Design review of the part built by this model. Coordinates are the model's own, in mm. A direction names the side the tool comes from. Coordinates: 2 decimals unless noted, no trailing zeros. Loops run counter-clockwise (first coordinate to the right, second up) from the corner with the lowest first, then second, coordinate; pieces in that order, holes last. Notation, with made-up numbers: M 34,23 L 75,23 A23 cw 75,34 Z; hole C 6.25,82 d5. An arc over 180 degrees is marked long. Put each result on its own line as item: value. Start each with the question number.
(1) For faces 4 (the cylindrical face through (28.795, 39.415, 2.535)), 5 (the flat face through (173.551, 4.735, 2.465)), list the 3-axis set-ups (+Z, -Z, +X, -X, +Y, -Y) from which the entire face can be reached by the end or side of a thin tool; tool diameter is ignored.
(2) Take a section at B-B, the plane x = 0. Give the boundary of the cut face in (y, z).
(3) Take a section at D-D, the plane y = 0. Give the boundary of the cut face in (x, z).
(4) Clearance check with flat-ended pins moving along their axes: pin 1 (2 mm diameter, centred on y = 5.5, z = 2.5, fed in from +X); pin 2 (1 mm diameter, centred on x = 27, z = 1, fed in from -Y); pin 3 (2.5 mm diameter, centred on x = 99.5, z = 2, fed in from -Y). State where each tip first meets the part, or that it passes through.
(5) Take a section at C-C, the plane y = 13.5. Give the boundary of the cut face in (x, z).
(6) Take a section at A-A, the plane z = 3.2. Give the boundary of the cut face in (x, y).
(7) The part is to be moulded in two halves that separate along Y. For faces 1 (the flat face through (97, 27, 0)), 2 (the cylindrical face through (-6.216, -6.495, 2.465)), 3 (the cylindrical face through (-3.309, 3.035, 2.465)), say which applies: +Y half, -Y half, draft (parallel to the pull), parting line (faces both ways), or undercut.
(8) For probe 1 along X at (y, z) = (-2, 1.05); probe 2 along Y at (x, z) = (137.5, 3.1); probe 3 along Y at (x, z) = (191, 2.25), list the stretches that pass through material, from the lowest coordinate up. Write a range as [from, to].
```python
from build123d import *

# Parameters (mm, degrees)
SKETCH1_R           = 4.49
BOSS_EXTRUDE1_DEPTH = 5
FILLET1_R           = 20
FILLET2_R           = 20
FILLET3_R           = 20
FILLET4_R           = 20


with BuildPart() as part:
    # Sketch1 → Boss-Extrude1 (new body)
    with BuildSketch(Plane.XY):
        with BuildLine():
            Line((-6.356889963, 6.356889963), (28.266220074, 40.98))
            Line((28.266220074, 40.98), (162.733779926, 40.98))
            Line((162.733779926, 40.98), (197.356889963, 6.356889963))
            ThreePointArc((197.356889963, 6.356889963), (197.356889963, -6.356889963), (184.643110037, -6.356889963))
            Line((184.643110037, -6.356889963), (156.286220074, 22))
            Line((156.286220074, 22), (34.713779926, 22))
            Line((34.713779926, 22), (6.356889963, -6.356889963))
            ThreePointArc((6.356889963, -6.356889963), (-6.356889963, -6.356889963), (-6.356889963, 6.356889963))
        make_face()
        Circle(SKETCH1_R, mode=Mode.SUBTRACT)
        with Locations((191, 0)):
            Circle(SKETCH1_R, mode=Mode.SUBTRACT)
    extrude(amount=BOSS_EXTRUDE1_DEPTH)

    # Fillet1
    fillet1_edges = [part.edges().sort_by_distance(p)[0] for p in [
        (28.266220074, 40.98, 2.5),
    ]]
    fillet(fillet1_edges, radius=FILLET1_R)

    # Fillet2
    fillet2_edges = [part.edges().sort_by_distance(p)[0] for p in [
        (34.713779926, 22, 2.5),
    ]]
    fillet(fillet2_edges, radius=FILLET2_R)

    # Fillet3
    fillet3_edges = [part.edges().sort_by_distance(p)[0] for p in [
        (162.733779926, 40.98, 2.5),
    ]]
    fillet(fillet3_edges, radius=FILLET3_R)

    # Fillet4
    fillet4_edges = [part.edges().sort_by_distance(p)[0] for p in [
        (156.286220074, 22, 2.5),
    ]]
    fillet(fillet4_edges, radius=FILLET4_R)


solid = part.part
```
Computed values:
1. face 4: +Z, -Z, -X, +Y
1. face 5: +Z, -Z, -Y
2. outline: M -8.99,0 L -4.49,0 L -4.49,5 L -8.99,5 Z; M 4.49,0 L 12.71,0 L 12.71,5 L 4.49,5 Z
3. outline: M -8.99,0 L -4.49,0 L -4.49,5 L -8.99,5 Z; M 4.49,0 L 12.71,0 L 12.71,5 L 4.49,5 Z; M 178.29,0 L 186.51,0 L 186.51,5 L 178.29,5 Z; M 195.49,0 L 199.99,0 L 199.99,5 L 195.49,5 Z
4. pin 1: stops at x = 198.78
4. pin 2: stops at y = 13.79
4. pin 3: stops at y = 22
5. outline: M 0.79,0 L 26.21,0 L 26.21,5 L 0.79,5 Z; M 164.79,0 L 190.21,0 L 190.21,5 L 164.79,5 Z
6. outline: M -6.36,6.36 A8.99 ccw 6.36,-6.36 L 28.86,16.14 A20 cw 43,22 L 148,22 A20 cw 162.14,16.14 L 184.64,-6.36 A8.99 ccw 197.36,6.36 L 168.59,35.12 A20 ccw 154.45,40.98 L 36.55,40.98 A20 ccw 22.41,35.12 Z; hole C 0,0 d8.98; hole C 191,0 d8.98
7. face 1: draft
7. face 2: parting line
7. face 3: undercut
8. probe 1: x = [-8.76, -4.02], [4.02, 10.71], [180.29, 186.98], [195.02, 199.76]
8. probe 2: y = [22, 40.98]
8. probe 3: y = [-8.99, -4.49], [4.49, 12.71]
